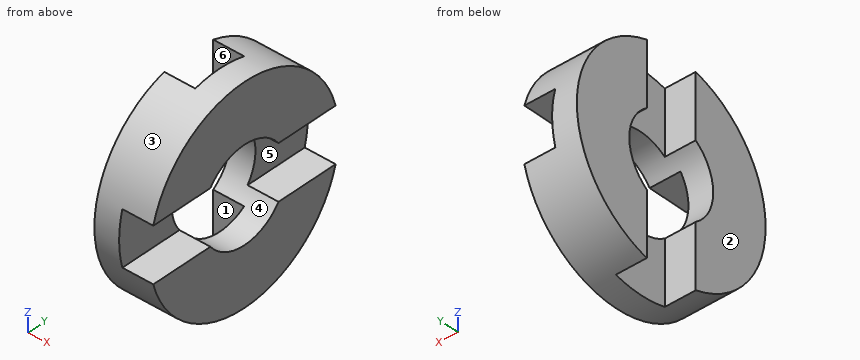
Autodesk Inventor part; units mm, degrees
ref_plane "C_XY" through (3.6, 0, 0) normal (1, 0, 0) x (0, 0, -1)
ref_plane "C_YZ" through (3.6, 0, 0) normal (0, 0, -1) x (0, 1, 0)
ref_plane "C_ZX" through (3.6, 0, 0) normal (0, 1, 0) x (1, 0, 0)
sketch "Sketch_1" plane through (0, 0, 0) normal (0, 0, 1) x (1, 0, 0)
  line L0 (7.2, 0) -> (0, 0)
  line L1 (0, 6) -> (7.2, 6)
  line L2 (7.2, 6) -> (7.2, 13.5)
  line L3 (7.2, 13.5) -> (0, 13.5)
  line L4 (0, 13.5) -> (0, 6)
revolve "Revolution1" add sketch "Sketch_1" angle 360 about axis through (7.2, 0, 0) along (1, 0, 0)
sketch "Sketch_2" plane through (0, 0, 0) normal (0, 0, 1) x (1, 0, 0)
  line L0 (0, 3.5) -> (0, -3.5)
  line L1 (0, -3.5) -> (4, -3.5)
  line L2 (4, -3.5) -> (4, 3.5)
  line L3 (4, 3.5) -> (0, 3.5)
extrude "Extrusion1" cut sketch "Sketch_2" along normal mid plane 27
sketch "Sketch_3" plane through (0, 0, 0) normal (0, 1, 0) x (-1, 0, 0)
  line L0 (-3.2, 3.5) -> (-7.2, 3.5)
  line L1 (-7.2, 3.5) -> (-7.2, -3.5)
  line L2 (-7.2, -3.5) -> (-3.2, -3.5)
  line L3 (-3.2, -3.5) -> (-3.2, 3.5)
extrude "Extrusion2" cut sketch "Sketch_3" along normal mid plane 27
ref_plane "C_XY" through (3.6, 0, 0) normal (1, 0, 0) x (0, 0, -1)
ref_plane "C_YZ" through (3.6, 0, 0) normal (0, 0, -1) x (0, 1, 0)
ref_plane "C_ZX" through (3.6, 0, 0) normal (0, 1, 0) x (1, 0, 0)
properties part number "MCOC_spacer26"
Here's how the part is built. I have some questions about the finished solid (model axes, mm). Face numbers are marked on the shaded views. A direction names the side the tool comes from. Give positions to 0.01 mm unless a question says otherwise; leave off trailing zeros. Loops run counter-clockwise (first coordinate to the right, second up) from the corner with the lowest first, then second, coordinate; pieces in that order, holes last. Notation, with made-up numbers: M 86,10.5 L 128,10.5 A23 cw 128,46.5 Z; hole C -7.75,3 d10. An arc over 180 degrees is marked long. Use one line per item in the form item = value. Start each with the question number.
Q1. Thinking about a two-plate mould opening in Y: for the marked faces 1, 2 and 3, which applies, +Y half, -Y half, draft (parallel to the pull), parting line (faces both ways), or undercut?
Q2. I need wall thicknesses on line 1 along Z through (x, y) = (5.25, -3.5); line 2 along X through (y, z) = (-10, -0.25); line 3 along X through (y, z) = (-1.75, 8.5). Which ranges of each line are inside material? Lowest first, please.
Q3. If we section it at C-C (z = -11.5): Write out the boundary of the cut face in (x, y).
Q4. If we section it at D-D (y = -11.5): Write out the boundary of the cut face in (x, z).
Q5. If we section it at A-A (z = 0): Write out the boundary of the cut face in (x, y).
Q6. Which directions (+Z, -Z, +X, -X, +Y, -Y) give clear straight access to the entire face, cutting with the end or side of a thin tool? Please do the marked faces 4, 5 and 6.
Q7. If we section it at B-B (x = 5.5): Write out the boundary of the cut face in (y, z).
Q8. Will these pins go through, and if not, where does the flat tip stop? pin 1 Ø2 at (x, y) = (6, 7) entering from -Z; pin 2 Ø3 at (x, y) = (2, 3.5) entering from -Z; pin 3 Ø3 at (x, z) = (2.5, -9) entering from -Y (3 decimals).
Taken from the geometry:
q1.face_1 = undercut
q1.face_2 = draft
q1.face_3 = parting line
q2.line_1 = -13.04 to -4.87, 4.87 to 13.04
q2.line_2 = 0 to 3.2
q2.line_3 = 4 to 7.2
q3.outline = M 0,-7.07 L 7.2,-7.07 L 7.2,7.07 L 0,7.07 L 0,3.5 L 4,3.5 L 4,-3.5 L 0,-3.5 Z
q4.outline = M 0,-7.07 L 7.2,-7.07 L 7.2,-3.5 L 3.2,-3.5 L 3.2,3.5 L 7.2,3.5 L 7.2,7.07 L 0,7.07 Z
q5.outline = M 0,-13.5 L 3.2,-13.5 L 3.2,-6 L 0,-6 Z; M 0,6 L 3.2,6 L 3.2,13.5 L 0,13.5 Z
q6.face_4 = +X, -X
q6.face_5 = +X, +Y, -Y
q6.face_6 = +Z, -Z, -X
q7.outline = M -13.04,-3.5 A13.5 ccw 13.04,-3.5 L 4.87,-3.5 A6 cw -4.87,-3.5 Z; M -13.04,3.5 L -4.87,3.5 A6 cw 4.87,3.5 L 13.04,3.5 A13.5 ccw Z
q8.pin_1 = -12.09
q8.pin_2 = -13.04
q8.pin_3 = -11.225
